Autodesk Inventor part; units mm, degrees
ref_plane "YZ Plane" through (0, 0, 0) normal (1, 0, 0) x (0, 1, 0)
ref_plane "XZ Plane" through (0, 0, 0) normal (0, 1, 0) x (-1, 0, 0)
ref_plane "XY Plane" through (0, 0, 0) normal (0, 0, 1) x (1, 0, 0)
ref_plane "Work Plane1" through (0, 0, 0) normal (0, 0, 1) x (1, 0, 0)
sketch "Sketch1" plane through (0, 0, 0) normal (0, 0, 1) x (1, 0, 0)
  arc A0 (-3.651, 13.5937) -> (-4.7619, 15.391) centre (-4.2064, 14.4923) ccw
  arc A1 (-3.651, 13.5937) -> (-6.4477, 10.2643) centre (0, 7.6875) ccw
  arc A2 (-8.4097, 11.0483) -> (-6.4477, 10.2643) centre (-7.4287, 10.6563) ccw
  arc A3 (-4.7619, 15.391) -> (-8.4097, 11.0483) centre (0, 7.6875) ccw
  arc A4 (6.4477, 10.2643) -> (8.4097, 11.0483) centre (7.4287, 10.6563) ccw
  arc A5 (6.4477, 10.2643) -> (3.651, 13.5937) centre (0, 7.6875) ccw
  arc A6 (4.7619, 15.391) -> (3.651, 13.5937) centre (4.2064, 14.4923) ccw
  arc A7 (8.4097, 11.0483) -> (4.7619, 15.391) centre (0, 7.6875) ccw
  arc A8 (-6.4563, 5.1322) -> (-8.4209, 4.3547) centre (-7.4386, 4.7434) ccw
  arc A9 (-6.4563, 5.1322) -> (-3.651, 1.7813) centre (0, 7.6875) ccw
  arc A10 (-4.7619, -0.016) -> (-3.651, 1.7813) centre (-4.2064, 0.8827) ccw
  arc A11 (-8.4209, 4.3547) -> (-4.7619, -0.016) centre (0, 7.6875) ccw
  arc A12 (3.651, 1.7813) -> (4.7619, -0.016) centre (4.2064, 0.8827) ccw
  arc A13 (3.651, 1.7813) -> (6.4563, 5.1322) centre (0, 7.6875) ccw
  arc A14 (8.4209, 4.3547) -> (6.4563, 5.1322) centre (7.4386, 4.7434) ccw
  arc A15 (4.7619, -0.016) -> (8.4209, 4.3547) centre (0, 7.6875) ccw
  circle A16 centre (10.65, 7.6999) radius 1.15
  circle A17 centre (0, 15.6875) radius 1.0564
  circle A18 centre (0, -0.3125) radius 1.0564
  circle A19 centre (0, 7.6875) radius 5
  circle A20 centre (0, 7.6875) radius 13.7
  line L0 (-116.625, -11.1875) -> (15.375, -11.1875)
  line L1 (15.375, -11.1875) -> (15.375, -7.6875)
  line L2 (-116.625, -7.6875) -> (15.375, -7.6875)
  line L3 (-116.625, -11.1875) -> (-116.625, -7.6875)
  line L4 (15.375, -7.6875) -> (-15.375, -7.6875)
  line L5 (-15.375, -7.6875) -> (-15.375, 22.3125)
  line L6 (-15.375, 22.3125) -> (15.375, 22.3125)
  line L7 (15.375, 22.3125) -> (15.375, -7.6875)
  circle A21 centre (0, 7.6875) radius 14.375
  circle A22 centre (0, 7.6875) radius 5.2
  arc A23 (-3.4406, 13.2535) -> (-4.9722, 15.7312) centre (-4.2064, 14.4923) ccw
  arc A24 (-3.4406, 13.2535) -> (-6.0763, 10.1158) centre (0, 7.6875) ccw
  arc A25 (-8.7812, 11.1968) -> (-6.0763, 10.1158) centre (-7.4287, 10.6563) ccw
  arc A26 (-4.9722, 15.7312) -> (-8.7812, 11.1968) centre (0, 7.6875) ccw
  arc A27 (4.9722, 15.7312) -> (3.4406, 13.2535) centre (4.2064, 14.4923) ccw
  arc A28 (6.0763, 10.1158) -> (3.4406, 13.2535) centre (0, 7.6875) ccw
  arc A29 (6.0763, 10.1158) -> (8.7812, 11.1968) centre (7.4287, 10.6563) ccw
  arc A30 (8.7812, 11.1968) -> (4.9722, 15.7312) centre (0, 7.6875) ccw
  arc A31 (3.4406, 2.1215) -> (6.0844, 5.2794) centre (0, 7.6875) ccw
  arc A32 (3.4406, 2.1215) -> (4.9722, -0.3562) centre (4.2064, 0.8827) ccw
  arc A33 (4.9722, -0.3562) -> (8.7928, 4.2075) centre (0, 7.6875) ccw
  arc A34 (8.7928, 4.2075) -> (6.0844, 5.2794) centre (7.4386, 4.7434) ccw
  arc A35 (-6.0844, 5.2794) -> (-8.7928, 4.2075) centre (-7.4386, 4.7434) ccw
  arc A36 (-6.0844, 5.2794) -> (-3.4406, 2.1215) centre (0, 7.6875) ccw
  arc A37 (-4.9722, -0.3562) -> (-3.4406, 2.1215) centre (-4.2064, 0.8827) ccw
  arc A38 (-8.7928, 4.2075) -> (-4.9722, -0.3562) centre (0, 7.6875) ccw
  circle A39 centre (10.65, 7.6999) radius 1.55
  point P0 (0, 0)
  dimension "d0" = 30
  dimension "d1" = 15.375
  dimension "d2" = 15.375
  dimension "d3" = 0.2
  dimension "d4" = 0.4
  dimension "d5" = 0.4
  dimension "d6" = 0.4
  dimension "d7" = 0.4
  dimension "d8" = 0.4
extrude "Extrusion1" add sketch "Sketch1" along normal blind 1 contours A20 | L2 L5 L6 L7 | A21
sketch "Sketch2" plane through (0, 0, 1) normal (0, 0, 1) x (1, 0, 0)
  line L0 (15.375, 22.3125) -> (-15.375, 22.3125)
  line L1 (-15.375, 22.3125) -> (-15.375, -7.6875)
  line L2 (-15.375, -7.6875) -> (15.375, -7.6875)
  line L3 (15.375, -7.6875) -> (15.375, 22.3125)
  circle A0 centre (0, 15.6875) radius 1.0564
  circle A1 centre (0, -0.3125) radius 1.0564
  circle A2 centre (0, 7.6875) radius 5.2
  arc A3 (-3.4406, 13.2535) -> (-6.0763, 10.1158) centre (0, 7.6875) ccw
  arc A4 (-8.7812, 11.1968) -> (-6.0763, 10.1158) centre (-7.4287, 10.6563) ccw
  arc A5 (-4.9722, 15.7312) -> (-8.7812, 11.1968) centre (0, 7.6875) ccw
  arc A6 (-3.4406, 13.2535) -> (-4.9722, 15.7312) centre (-4.2064, 14.4923) ccw
  arc A7 (6.0763, 10.1158) -> (3.4406, 13.2535) centre (0, 7.6875) ccw
  arc A8 (4.9722, 15.7312) -> (3.4406, 13.2535) centre (4.2064, 14.4923) ccw
  arc A9 (8.7812, 11.1968) -> (4.9722, 15.7312) centre (0, 7.6875) ccw
  arc A10 (6.0763, 10.1158) -> (8.7812, 11.1968) centre (7.4287, 10.6563) ccw
  arc A11 (3.4406, 2.1215) -> (4.9722, -0.3562) centre (4.2064, 0.8827) ccw
  arc A12 (3.4406, 2.1215) -> (6.0844, 5.2794) centre (0, 7.6875) ccw
  arc A13 (8.7928, 4.2075) -> (6.0844, 5.2794) centre (7.4386, 4.7434) ccw
  arc A14 (4.9722, -0.3562) -> (8.7928, 4.2075) centre (0, 7.6875) ccw
  arc A15 (-6.0844, 5.2794) -> (-3.4406, 2.1215) centre (0, 7.6875) ccw
  arc A16 (-4.9722, -0.3562) -> (-3.4406, 2.1215) centre (-4.2064, 0.8827) ccw
  arc A17 (-8.7928, 4.2075) -> (-4.9722, -0.3562) centre (0, 7.6875) ccw
  arc A18 (-6.0844, 5.2794) -> (-8.7928, 4.2075) centre (-7.4386, 4.7434) ccw
  circle A19 centre (10.65, 7.6999) radius 1.55
  arc A20 (4.9722, 15.7312) -> (3.4406, 13.2535) centre (4.2064, 14.4923) ccw
  line L4 (4.2064, 15.9488) -> (15.375, 15.9488)
  line L5 (15.375, -7.6875) -> (15.375, 22.3125)
  line L6 (4.2064, -0.5738) -> (15.375, -0.5738)
  arc A21 (6.0763, 10.1158) -> (8.7812, 11.1968) centre (7.4287, 10.6563) ccw
  line L7 (6.0763, 10.1158) -> (6.0844, 5.2794)
  point P0 (0, 0)
extrude "Extrusion2" add sketch "Sketch2" along normal blind 1.5 contours L3 L4 A8 A7 L7 A12 A11 L6 L2 L1 L0
sketch "Sketch3" plane through (0, 0, 2.5) normal (0, 0, 1) x (1, 0, 0)
  line L0 (15.375, -7.6875) -> (15.375, -0.5738)
  line L1 (15.375, -0.5738) -> (4.2064, -0.5738)
  arc A0 (3.4406, 2.1215) -> (4.2064, -0.5738) centre (4.2064, 0.8827) ccw
  arc A1 (3.4406, 2.1215) -> (6.0844, 5.2794) centre (0, 7.6875) ccw
  line L2 (6.0844, 5.2794) -> (6.0763, 10.1158)
  arc A2 (6.0763, 10.1158) -> (3.4406, 13.2535) centre (0, 7.6875) ccw
  arc A3 (4.2064, 15.9488) -> (3.4406, 13.2535) centre (4.2064, 14.4923) ccw
  line L3 (4.2064, 15.9488) -> (15.375, 15.9488)
  line L4 (15.375, 15.9488) -> (15.375, 22.3125)
  line L5 (15.375, 22.3125) -> (-15.375, 22.3125)
  line L6 (-15.375, 22.3125) -> (-15.375, -7.6875)
  line L7 (-15.375, -7.6875) -> (15.375, -7.6875)
  circle A4 centre (0, 15.6875) radius 1.0564
  circle A5 centre (0, -0.3125) radius 1.0564
  arc A6 (-6.0844, 5.2794) -> (-8.7928, 4.2075) centre (-7.4386, 4.7434) ccw
  arc A7 (-6.0844, 5.2794) -> (-3.4406, 2.1215) centre (0, 7.6875) ccw
  arc A8 (-4.9722, -0.3562) -> (-3.4406, 2.1215) centre (-4.2064, 0.8827) ccw
  arc A9 (-8.7928, 4.2075) -> (-4.9722, -0.3562) centre (0, 7.6875) ccw
  arc A10 (-3.4406, 13.2535) -> (-4.9722, 15.7312) centre (-4.2064, 14.4923) ccw
  arc A11 (-3.4406, 13.2535) -> (-6.0763, 10.1158) centre (0, 7.6875) ccw
  arc A12 (-8.7812, 11.1968) -> (-6.0763, 10.1158) centre (-7.4287, 10.6563) ccw
  arc A13 (-4.9722, 15.7312) -> (-8.7812, 11.1968) centre (0, 7.6875) ccw
  circle A14 centre (0, 7.6875) radius 5.2
  circle A15 centre (0, 15.6875) radius 2.65
  circle A16 centre (0, -0.3125) radius 1.0564
  circle A17 centre (0, -0.3125) radius 2.65
  arc A18 (-2.4425, 10.6818) -> (-4.3563, 11.5819) centre (-5.3868, 6.906) ccw
  arc A19 (-4.3563, 11.5819) -> (-4.9119, 10.8525) centre (0, 7.6875) ccw
  arc A20 (-4.9119, 10.8525) -> (-3.5356, 9.2466) centre (-0.678, 13.0883) ccw
  arc A21 (-3.5356, 9.2466) -> (-3.736, 8.6743) centre (0, 7.6875) ccw
  arc A22 (-3.736, 8.6743) -> (-5.8134, 8.2775) centre (-3.8987, 3.889) ccw
  arc A23 (-5.8134, 8.2775) -> (-5.8341, 7.3609) centre (0, 7.6875) ccw
  arc A24 (-5.8341, 7.3609) -> (-3.7768, 6.8706) centre (-3.723, 11.6584) ccw
  arc A25 (-3.7768, 6.8706) -> (-3.6025, 6.2899) centre (0, 7.6875) ccw
  arc A26 (-3.6025, 6.2899) -> (-5.05, 4.7478) centre (-0.9214, 2.3228) ccw
  arc A27 (-5.05, 4.7478) -> (-4.5279, 3.994) centre (0, 7.6875) ccw
  arc A28 (-4.5279, 3.994) -> (-2.5753, 4.8067) centre (-5.346, 8.7117) ccw
  arc A29 (-2.5753, 4.8067) -> (-2.093, 4.4393) centre (0, 7.6875) ccw
  arc A30 (-2.093, 4.4393) -> (-2.3576, 2.341) centre (2.4078, 2.8058) ccw
  arc A31 (-2.3576, 2.341) -> (-1.4922, 2.038) centre (0, 7.6875) ccw
  arc A32 (-1.4922, 2.038) -> (-0.3902, 3.8431) centre (-4.927, 5.3738) ccw
  arc A33 (-0.3902, 3.8431) -> (0.216, 3.8294) centre (0, 7.6875) ccw
  arc A34 (0.216, 3.8294) -> (1.2353, 1.9763) centre (4.8174, 5.1534) ccw
  arc A35 (1.2353, 1.9763) -> (2.1135, 2.2398) centre (0, 7.6875) ccw
  arc A36 (2.1135, 2.2398) -> (1.944, 4.348) centre (-2.6261, 2.9196) ccw
  arc A37 (1.944, 4.348) -> (2.4425, 4.6932) centre (0, 7.6875) ccw
  arc A38 (2.4425, 4.6932) -> (4.3563, 3.7931) centre (5.3868, 8.469) ccw
  arc A39 (4.3563, 3.7931) -> (4.9119, 4.5225) centre (0, 7.6875) ccw
  arc A40 (4.9119, 4.5225) -> (3.5356, 6.1284) centre (0.678, 2.2867) ccw
  arc A41 (3.5356, 6.1284) -> (3.736, 6.7007) centre (0, 7.6875) ccw
  arc A42 (3.736, 6.7007) -> (5.8134, 7.0975) centre (3.8987, 11.486) ccw
  arc A43 (5.8134, 7.0975) -> (5.8341, 8.0141) centre (0, 7.6875) ccw
  arc A44 (5.8341, 8.0141) -> (3.7768, 8.5044) centre (3.723, 3.7166) ccw
  arc A45 (3.7768, 8.5044) -> (3.6025, 9.0851) centre (0, 7.6875) ccw
  arc A46 (3.6025, 9.0851) -> (5.05, 10.6272) centre (0.9214, 13.0522) ccw
  arc A47 (5.05, 10.6272) -> (4.5279, 11.381) centre (0, 7.6875) ccw
  arc A48 (4.5279, 11.381) -> (2.5753, 10.5683) centre (5.346, 6.6633) ccw
  arc A49 (2.5753, 10.5683) -> (2.093, 10.9357) centre (0, 7.6875) ccw
  arc A50 (2.093, 10.9357) -> (2.3576, 13.034) centre (-2.4078, 12.5692) ccw
  arc A51 (2.3576, 13.034) -> (1.4922, 13.337) centre (0, 7.6875) ccw
  arc A52 (1.4922, 13.337) -> (0.3902, 11.5319) centre (4.927, 10.0012) ccw
  arc A53 (0.3902, 11.5319) -> (-0.216, 11.5456) centre (0, 7.6875) ccw
  arc A54 (-0.216, 11.5456) -> (-1.2353, 13.3987) centre (-4.8174, 10.2216) ccw
  arc A55 (-1.2353, 13.3987) -> (-2.1135, 13.1352) centre (0, 7.6875) ccw
  arc A56 (-2.1135, 13.1352) -> (-1.944, 11.027) centre (2.6261, 12.4554) ccw
  arc A57 (-1.944, 11.027) -> (-2.4425, 10.6818) centre (0, 7.6875) ccw
  circle A58 centre (0, 7.6875) radius 5.8433
  circle A59 centre (0, 7.6875) radius 6.5436
  arc A60 (-3.4406, 13.2535) -> (-4.9722, 15.7312) centre (-4.2064, 14.4923) ccw
  line L8 (-2.9676, 15.2581) -> (-2.615, 15.2581)
  arc A61 (4.9722, 15.7312) -> (3.4406, 13.2535) centre (4.2064, 14.4923) ccw
  line L9 (2.9676, 15.2581) -> (2.615, 15.2581)
  arc A62 (3.4406, 2.1215) -> (4.9722, -0.3562) centre (4.2064, 0.8827) ccw
  line L10 (2.8055, 0.4846) -> (2.5273, 0.4846)
  arc A63 (-4.9722, -0.3562) -> (-3.4406, 2.1215) centre (-4.2064, 0.8827) ccw
  line L11 (-2.8055, 0.4846) -> (-2.5273, 0.4846)
  arc A64 (-8.7812, 11.1968) -> (-6.0763, 10.1158) centre (-7.4287, 10.6563) ccw
  line L12 (-7.7556, 9.237) -> (-7.7556, 6.165)
  point P0 (0, 0)
  point P1 (-6.0844, 5.2794)
  point P2 (-6.0763, 10.1158)
  point P3 (2.9676, 15.2581)
  dimension "d13" = 5.3
  dimension "d14" = 5.3
extrude "Extrusion3" add sketch "Sketch3" along normal blind 1 contours L7 L6 L5 L4 L3 A3 L9 A15 L8 A10 A13 A12 L12 A6 A9 A8 L11 A17 L10 A0 L1 L0
equation "\"d2\" = d1"
properties part number "front_motur_holder"
Part model, mm, in its own coordinate system. A direction names the side the tool comes from. Round coordinates to 2 decimals unless told otherwise and drop trailing zeros. Loops run counter-clockwise (first coordinate to the right, second up) from the corner with the lowest first, then second, coordinate; pieces in that order, holes last. Notation, with made-up numbers: (-9.75, -37.5) - (30.25, -37.5) arc R29 ccw to (30.25, -5.5) - close; hole circle Ø11 at (-38, 60.5). An arc over 180 degrees is marked (long way). Answer as a JSON object with one key per item and string values.
Item 1: Wall check: L1, parallel to Y at x = 0, z = 1.5; L2, parallel to Y at x = 10.65, z = 0.85; L3, parallel to Y at x = -6.5, z = 0.6. Give the ranges that are in metal, low to high.
Output:
{"L1": "-7.69 to -1.37, 0.74 to 2.49, 12.89 to 14.63, 16.74 to 22.31", "L2": "-7.69 to 6.15, 9.25 to 22.31", "L3": "-7.69 to 0.82, 5.86 to 9.53, 14.56 to 22.31"}
Item 2: Band-saw the part on A-A on x = 0. List the corners of the cut face in (y, z).
Output:
{"outline": "(-7.69, 0) - (-1.37, 0) - (-1.37, 2.5) - (-2.96, 2.5) - (-2.96, 3.5) - (-7.69, 3.5) - close; (0.74, 0) - (2.49, 0) - (2.49, 2.5) - (0.74, 2.5) - close; (12.89, 0) - (14.63, 0) - (14.63, 2.5) - (12.89, 2.5) - close; (16.74, 0) - (22.31, 0) - (22.31, 3.5) - (18.34, 3.5) - (18.34, 2.5) - (16.74, 2.5) - close"}
Item 3: Pull direction X, two halves, no side cores. Call faces 6 (the face through (11, 10, 1)), 7 (the face through (3.34, -0.29, 2.99)), 8 (the face through (7.999, 9.316, 0.493)), 9 (the face through (-15.375, 8, 2)): pulls with the +X half, pulls with the -X half, needs draft (parallel to the pull), parting line crosses it, or undercut.
Output:
{"face 6": "needs draft", "face 7": "pulls with the +X half", "face 8": "undercut", "face 9": "pulls with the -X half"}
Item 4: Band-saw the part on C-C on z = 0.55. State how many separate pieces and enclosed holes the cut face has, plus the area to 3 significant figures.
Output:
{"separate pieces": "1", "enclosed holes": "8", "area": "737 mm2"}
Item 5: Band-saw the part on B-B on x = 10.65. List the corners of the cut face in (y, z).
Output:
{"outline": "(-7.69, 0) - (6.15, 0) - (6.15, 1) - (-0.57, 1) - (-0.57, 3.5) - (-7.69, 3.5) - close; (9.25, 0) - (22.31, 0) - (22.31, 3.5) - (15.95, 3.5) - (15.95, 1) - (9.25, 1) - close"}
Item 6: Pin check, flat tips, straight feed: pin 1 (7 mm diameter, centred on x = -2, y = 6, fed in from +Z); pin 2 (8.5 mm diameter, centred on x = 0, y = 7.69, fed in from -Z); pin 3 (1.1 mm diameter, centred on y = 7, z = 3, fed in from +X); pin 4 (3.5 mm diameter, centred on x = 9.5, y = 6.5, fed in from +Z). Stop position of each tip, or through.
Output:
{"pin 1": "z = 2.5", "pin 2": "through", "pin 3": "x = 6.08", "pin 4": "z = 1"}
Item 7: Tool access for faces 1 (the face through (0, -7.688, 2)), 2 (the face through (10, -0.574, 2)), 3 (the face through (0, 22.312, 2)), 4 (the face through (4.99, 11.92, 1.23)), 5 (the face through (-0.064, 18.337, 2.993)): list every direction of +Z, -Z, +X, -X, +Y, -Y with a clear straight run to the whole face (end or side of a thin tool).
Output:
{"face 1": "+Z, -Z, +X, -X, -Y", "face 2": "+Z, +X", "face 3": "+Z, -Z, +X, -X, +Y", "face 4": "+Z, -Z", "face 5": "+Z"}
